Check sheet for the modelled part. Datum: model origin and axes. Units: mm. A direction names the side the tool comes from. Coordinates: 2 decimals unless noted, no trailing zeros. Loops run counter-clockwise (first coordinate to the right, second up) from the corner with the lowest first, then second, coordinate; pieces in that order, holes last. Notation, with made-up numbers: M 19.25,78 L 70.25,78 A18 cw 70.25,89 Z; hole C 80.5,-23.75 d9. An arc over 180 degrees is marked long. Write each question's results on one line, items separated by ' | '. Start each with the question number.
Autodesk Fusion 360 part; units mm, degrees
sketch "Sketch1" plane through (0, 0, 0) normal (0, 0, 1) x (1, 0, 0)
  line L0 (17.85, 0) -> (24.15, 0)
  line L1 (24.15, -8) -> (17.85, -13.9)
  line L2 (17.85, 8) -> (17.85, 0)
  line L3 (17.85, -13.9) -> (17.85, 13.9)
  line L4 (17.85, -8) -> (17.85, 0)
  line L5 (17.85, 0) -> (24.15, 0)
  line L6 (17.85, 13.9) -> (-24.15, 13.9)
  line L7 (24.15, 0) -> (24.15, -8)
  line L8 (-24.15, 13.9) -> (24.15, -13.9) construction
  line L9 (24.15, 8) -> (23.8007, 8)
  line L10 (24.15, -8) -> (17.85, -8)
  line L11 (24.15, 8) -> (17.85, 8)
  line L12 (24.15, 0) -> (24.15, 8)
  line L13 (17.85, 13.9) -> (24.15, 8)
  line L14 (-24.15, 13.9) -> (24.15, 13.9)
  line L15 (24.15, 13.9) -> (24.15, -13.9)
  line L16 (24.15, -13.9) -> (-24.15, -13.9)
  line L17 (-24.15, -13.9) -> (-24.15, 13.9)
  line L18 (24.15, 13.9) -> (-24.15, -13.9) construction
  line L19 (60, -20) -> (-40, -20)
  line L20 (-40, -20) -> (-40, 20)
  line L21 (-40, 20) -> (60, 20)
  line L22 (60, 20) -> (60, -20)
  line L23 (60, 20) -> (50, 20)
  line L24 (50, 20) -> (50, 17)
  line L25 (50, 17) -> (60, 17)
  line L26 (60, 17) -> (60, 20)
  line L27 (60, -20) -> (50, -20)
  line L28 (50, -20) -> (50, -17)
  line L29 (50, -17) -> (60, -17)
  line L30 (60, -17) -> (60, -20)
  line L31 (-40, -20) -> (-30, -20)
  line L32 (-30, -20) -> (-30, -17)
  line L33 (-30, -17) -> (-40, -17)
  line L34 (-40, -17) -> (-40, -20)
  line L35 (-40, 20) -> (-30, 20)
  line L36 (-30, 20) -> (-30, 17)
  line L37 (-30, 17) -> (-40, 17)
  line L38 (-40, 17) -> (-40, 20)
  dimension "d1" = 48.3
  dimension "d2" = 27.8
  dimension "d3" = 42
  dimension "d4" = 8
  dimension "d5" = 8
  dimension "d6" = 100
  dimension "d7" = 40
  dimension "d8" = 3
  dimension "d9" = 10
  dimension "d10" = 10
  dimension "d11" = 3
  dimension "d12" = 3
  dimension "d13" = 10
  dimension "d14" = 10
  dimension "d15" = 3
  dimension "d25" = 6.1
  dimension "d26" = 15.85
extrude "Extrude1" add sketch "Sketch1" along normal blind 3 contours L1 L15 L16 | L13 L14 L15 | L19 L22 L27 L28 L29 L30 | L19 L20 L21 L22 L24 L25 L28 L29 L32 L33 L36 L37 | L19 L20 L31 L32 L33 L34 | L21 L22 L23 L24 L25 L26 | L20 L21 L35 L36 L37 L38
extrude "Extrude2" add sketch "Sketch1" against normal blind 17 contours L19 L22 L27 L28 L29 L30 | L19 L20 L31 L32 L33 L34 | L21 L22 L23 L24 L25 L26 | L20 L21 L35 L36 L37 L38
sketch "Sketch2" plane through (0, 20, 0) normal (0, 1, 0) x (-1, 0, 0)
  line L0 (-50, 0) -> (30, 0)
  line L1 (30, 0) -> (30, -17)
  line L2 (30, -17) -> (40, -17)
  line L3 (40, -17) -> (40, 3)
  line L4 (40, 3) -> (-60, 3)
  line L5 (-60, 3) -> (-60, -17)
  line L6 (-60, -17) -> (-50, -17)
  line L7 (-50, -17) -> (-50, 0)
  circle A0 centre (35, -7) radius 1.625
  circle A1 centre (-55, -7) radius 1.625
  dimension "d20" = 3.25
  dimension "d21" = 3.25
  dimension "d27" = 5
extrude "Extrude3" cut sketch "Sketch2" against normal up to surface (40 mm away) contours A0 | A1
chamfer "Chamfer1" distance 3 angle 45 8 edges at (-35, -17, 0) (-35, 17, 0) (55, -17, 0) (55, 17, 0) (50, 18.5, 0) (50, -18.5, 0) (-30, -18.5, 0) (-30, 18.5, 0)
1) Set-up check for faces 4 (the flat face through (-35, -17, -10)), 5 (the flat face through (49, -18, -2)), 6 (the flat face through (-3, 13.9, 1)): record each of +Z, -Z, +X, -X, +Y, -Y from which the full face is reachable in a straight line by a thin tool's end or side.
2) Section check D-D (y = -5). Enter the section's corners in (x, z).
3) Section check A-A (z = -7). Give the number of separate pieces and of enclosed holes in the cut face, then the cut area to 3 significant figures.
4) Thickness scan on probe 1 along Z at (x, y) = (-35, -19) (3 decimals); probe 2 along Z at (x, y) = (30.5, 10). Record the ranges inside material, lowest first.
5) Release check for a two-part mould opening along X. For faces 1 (the flat face through (50, -19, -10)), 2 (the flat face through (-34, 16, -2)), 3 (the cylindrical face through (-33.377, 18.521, -6.929)) record: +X half, -X half, draft (parallel to the pull), parting line (faces both ways), or undercut.
6) Section check C-C (x = -35). Enter the section's corners in (y, z) (3 decimals), then the cut area to 4 significant figures.
7) Section check B-B (z = -12.25). Enter the section's corners in (x, y), then the cut area to 3 significant figures.
8) Gauge pin test, flat ends, axial feed: P1, Ø4, axis at x = -35, z = -7, coming from the -Y side; P2, Ø5, axis at x = 26, y = -10, coming from the -Z side. Record the tip position at first contact, or that the pin passes through.
Return value:
1) face 4: -Z, +X, -X | face 5: -Z, +Y, -Y | face 6: +Z, -Z
2) outline: M -40,0 L -24.15,0 L -24.15,3 L -40,3 Z; M 24.15,0 L 60,0 L 60,3 L 24.15,3 Z
3) separate pieces: 8 | enclosed holes: 0 | area: 81.0 mm2
4) probe 1: z = -17 to -8.625, -5.375 to 3 | probe 2: z = 0 to 3
5) face 1: undercut | face 2: draft | face 3: undercut
6) outline: M -20,-17 L -17,-17 L -17,-8.625 L -20,-8.625 Z; M -20,-5.375 L -17,-5.375 L -17,-3 L -14,0 L 14,0 L 17,-3 L 17,-5.375 L 20,-5.375 L 20,3 L -20,3 Z; M 17,-17 L 20,-17 L 20,-8.625 L 17,-8.625 Z | area: 211.5 mm2
7) outline: M -40,-20 L -30,-20 L -30,-17 L -40,-17 Z; M -40,17 L -30,17 L -30,20 L -40,20 Z; M 50,-20 L 60,-20 L 60,-17 L 50,-17 Z; M 50,17 L 60,17 L 60,20 L 50,20 Z | area: 120 mm2
8) P1: stops at y = -20 | P2: stops at z = 0
